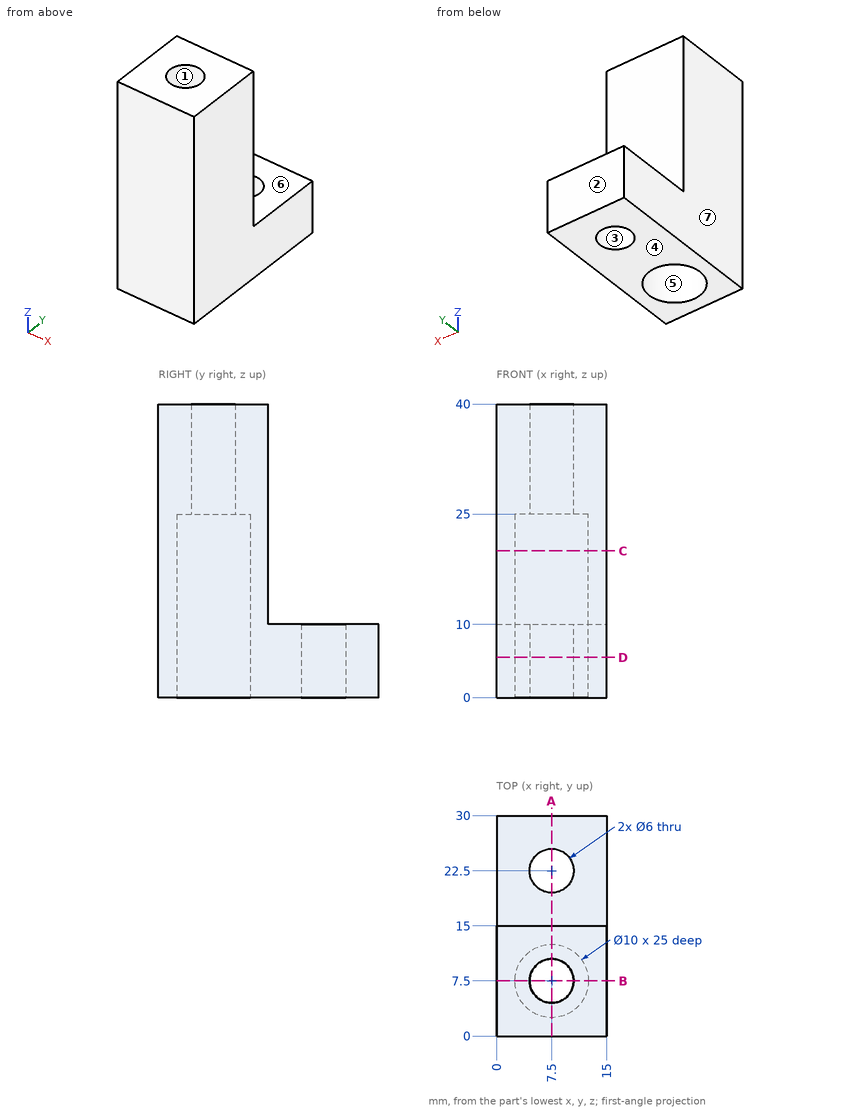
Source: three-view drawing plus pictorial views. Frame: mm from the lowest corner of the part. A direction names the side the tool comes from. Coordinates: 2 decimals unless noted, no trailing zeros. Order: outer loops, then holes, each group sorted by start corner. A loop starts at its lowest first (then second) coordinate and runs counter-clockwise, first axis right, second up.
Item 1: Cut plane C-C (z = 20). Return loops of the section in (x, y), plus the area to 3 significant figures.
Output values:
outline: (0, 0) - (15, 0) - (15, 15) - (0, 15) - close; hole circle Ø10 at (7.5, 7.5)
area: 146 mm2
Item 2: Cut plane B-B (y = 7.5). Return loops of the section in (x, z).
Output values:
outline: (0, 0) - (2.5, 0) - (2.5, 25) - (4.5, 25) - (4.5, 40) - (0, 40) - close; (10.5, 25) - (12.5, 25) - (12.5, 0) - (15, 0) - (15, 40) - (10.5, 40) - close
Item 3: Set-up query: the marked faces 5, 6 and 7. Return all of +Z, -Z, +X, -X, +Y, -Y with unobstructed straight access to the full face (end or side cutting, diameter ignored); none if empty.
Output values:
face 5: -Z
face 6: +Z, +X, -X, +Y
face 7: +Z, -Z, -X, +Y, -Y
Item 4: Cut plane D-D (z = 5.5). Return loops of the section in (x, y), plus the area to 3 significant figures.
Output values:
outline: (0, 0) - (15, 0) - (15, 30) - (0, 30) - close; hole circle Ø10 at (7.5, 7.5); hole circle Ø6 at (7.5, 22.5)
area: 343 mm2
Item 5: Material intervals for line 1 (Y direction, x = 7.5, z = 4.5); line 2 (Y direction, x = 7.5, z = 33.5); line 3 (X direction, y = 7.5, z = 17.75), sorted ascending.
Output values:
line 1: y = 0 to 2.5, 12.5 to 19.5, 25.5 to 30
line 2: y = 0 to 4.5, 10.5 to 15
line 3: x = 0 to 2.5, 12.5 to 15
Item 6: First-contact query: P1, Ø3, axis at x = 9.5, y = 10, coming from the -Z side; P2, Ø1, axis at x = 13, z = 33, coming from the +Y side; P3, Ø7.5, axis at x = 7, y = 26, coming from the +Z side. Flat tips, straight axial feed; report the tip coordinate or a pass-through.
Output values:
P1: stops at z = 25
P2: stops at y = 15
P3: stops at z = 10
Item 7: Cut plane A-A (x = 7.5). Return loops of the section in (y, z).
Output values:
outline: (0, 0) - (2.5, 0) - (2.5, 25) - (4.5, 25) - (4.5, 40) - (0, 40) - close; (10.5, 25) - (12.5, 25) - (12.5, 0) - (19.5, 0) - (19.5, 10) - (15, 10) - (15, 40) - (10.5, 40) - close; (25.5, 0) - (30, 0) - (30, 10) - (25.5, 10) - close
Item 8: Pull-direction query (Y, two-part tool) for the marked faces 1, 2, 3 and 4; classes: pulls with the +Y half, pulls with the -Y half, needs draft (parallel to the pull), parting line crosses it, or undercut.
Output values:
face 1: undercut
face 2: pulls with the +Y half
face 3: undercut
face 4: needs draft
